```python
from build123d import *

# Parameters (mm, degrees)
SKETCH1_W                        = 82.55
SKETCH1_H                        = 127
EXTRUDE1_DEPTH                   = 12.7
SKETCH2_W                        = 57.15
SKETCH2_H                        = 127
CUT_EXTRUDE1_DEPTH               = 1.016
CUT_EXTRUDE2_REACH               = 14.7
SKETCH4_W                        = 12.7
SKETCH4_H                        = 127
EXTRUDE3_DEPTH                   = 107.95
EXTRUDE4_DEPTH                   = 12.7
CUT_EXTRUDE3_REACH               = 97.25
CUT_EXTRUDE4_DEPTH               = 96.25
F_1_2_13_TAPPED_HOLE1_AT_2_COUNT = 2
F_1_2_13_TAPPED_HOLE1_AT_2_PITCH = 34.925
F_1_2_13_TAPPED_HOLE2_AT_2_COUNT = 2
F_1_2_13_TAPPED_HOLE2_AT_2_PITCH = 44.45
FILLET1_R                        = 6.35
F_1_2_13_TAPPED_HOLE3_AT_2_COUNT = 2
F_1_2_13_TAPPED_HOLE3_AT_2_PITCH = 34.925
F_1_2_13_TAPPED_HOLE4_AT_2_COUNT = 2
F_1_2_13_TAPPED_HOLE4_AT_2_PITCH = 44.45


with BuildPart() as part:
    # Sketch1 → Extrude1 (new body)
    with BuildSketch(Plane.XY):
        with Locations((-41.275, 63.5)):
            Rectangle(SKETCH1_W, SKETCH1_H)
    extrude(amount=EXTRUDE1_DEPTH)

    # Sketch2 → Cut-Extrude1 (cut)
    with BuildSketch(Plane(origin=(0, 0, 0), x_dir=(-1, 0, 0), z_dir=(0, 0, -1))):
        with Locations((41.275, 63.5)):
            Rectangle(SKETCH2_W, SKETCH2_H)
    extrude(amount=-CUT_EXTRUDE1_DEPTH, mode=Mode.SUBTRACT)

    # Sketch3 → Cut-Extrude2 (cut, up to next)
    with BuildSketch(Plane.XY.offset(12.7), mode=Mode.PRIVATE) as cut_extrude2_sk1:
        with BuildLine():
            Line((-47.625, 114.935), (-34.925, 114.935))
            ThreePointArc((-34.925, 114.935), (-25.4, 105.41), (-34.925, 95.885))
            Line((-34.925, 95.885), (-47.625, 95.885))
            ThreePointArc((-47.625, 95.885), (-57.15, 105.41), (-47.625, 114.935))
        make_face()
    cut_extrude2_tool1 = extrude(cut_extrude2_sk1.sketch, amount=-CUT_EXTRUDE2_REACH, mode=Mode.PRIVATE) & part.part
    add(cut_extrude2_tool1.solids().sort_by_distance((-41.275, 105.41, 12.7))[0], mode=Mode.SUBTRACT)
    # Sketch3 → Cut-Extrude2 (cut, up to next)
    with BuildSketch(Plane.XY.offset(12.7), mode=Mode.PRIVATE) as cut_extrude2_sk2:
        with BuildLine():
            Line((-47.625, 31.115), (-34.925, 31.115))
            ThreePointArc((-34.925, 31.115), (-25.4, 21.59), (-34.925, 12.065))
            Line((-34.925, 12.065), (-47.625, 12.065))
            ThreePointArc((-47.625, 12.065), (-57.15, 21.59), (-47.625, 31.115))
        make_face()
    cut_extrude2_tool2 = extrude(cut_extrude2_sk2.sketch, amount=-CUT_EXTRUDE2_REACH, mode=Mode.PRIVATE) & part.part
    add(cut_extrude2_tool2.solids().sort_by_distance((-41.275, 21.59, 12.7))[0], mode=Mode.SUBTRACT)
    # Sketch3 → Cut-Extrude2 (cut, up to next)
    with BuildSketch(Plane.XY.offset(12.7), mode=Mode.PRIVATE) as cut_extrude2_sk3:
        with BuildLine():
            Line((-47.625, 76.835), (-34.925, 76.835))
            ThreePointArc((-34.925, 76.835), (-25.4, 67.31), (-34.925, 57.785))
            Line((-34.925, 57.785), (-47.625, 57.785))
            ThreePointArc((-47.625, 57.785), (-57.15, 67.31), (-47.625, 76.835))
        make_face()
    cut_extrude2_tool3 = extrude(cut_extrude2_sk3.sketch, amount=-CUT_EXTRUDE2_REACH, mode=Mode.PRIVATE) & part.part
    add(cut_extrude2_tool3.solids().sort_by_distance((-41.275, 67.31, 12.7))[0], mode=Mode.SUBTRACT)

    # Sketch4 → Extrude3 (add)
    with BuildSketch(Plane.XY.offset(12.7)):
        with Locations((-6.35, 63.5)):
            Rectangle(SKETCH4_W, SKETCH4_H)
    extrude(amount=EXTRUDE3_DEPTH)

    # Sketch5 → Extrude4 (add)
    with BuildSketch(Plane(origin=(0, 0, 0), x_dir=(0, 0, -1), z_dir=(1, 0, 0))):
        with BuildLine():
            Line((-120.65, 0), (-44.45, 0))
            Line((-44.45, 0), (-44.45, 299.085))
            Line((-44.45, 299.085), (-184.277, 299.085))
            Line((-184.277, 299.085), (-184.277, 149.86))
            Line((-184.277, 149.86), (-133.35, 149.86))
            ThreePointArc((-133.35, 149.86), (-124.369743879, 146.140256121), (-120.65, 137.16))
            Line((-120.65, 137.16), (-120.65, 0))
        make_face()
    extrude(amount=EXTRUDE4_DEPTH)

    # Sketch6 → Cut-Extrude3 (cut, up to next)
    with BuildSketch(Plane(origin=(12.7, 0, 0), x_dir=(0, 0, -1), z_dir=(1, 0, 0)), mode=Mode.PRIVATE) as cut_extrude3_sk1:
        Polygon((-127.127, 299.085), (-44.45, 127.635), (-44.45, 299.085), align=None)
    cut_extrude3_tool1 = extrude(cut_extrude3_sk1.sketch, amount=-CUT_EXTRUDE3_REACH, mode=Mode.PRIVATE) & part.part
    add(cut_extrude3_tool1.solids().sort_by_distance((12.7, 241.935, 72.009))[0], mode=Mode.SUBTRACT)

    # Sketch7 → Cut-Extrude4 (cut, through all)
    with BuildSketch(Plane(origin=(12.7, 0, 0), x_dir=(0, 0, -1), z_dir=(1, 0, 0))):
        Polygon((-184.277, 149.86), (-144.469555556, 149.86), (-184.277, 232.41), align=None)
    extrude(amount=-CUT_EXTRUDE4_DEPTH, mode=Mode.SUBTRACT)

    # Sketch8 → 1/2-13 Tapped Hole1 (revolve, cut)
    with BuildSketch(Plane(origin=(12.7, 248.285, 155.702), x_dir=(0, 0, -1), z_dir=(0, 1, 0))):
        Polygon((0, 0), (0, 12.7), (6.985, 12.7), (5.35813, 10.828500149), (5.35813, 1.871499851), (6.985, 0), align=None)
    f_1_2_13_tapped_hole1 = revolve(axis=Axis((19.05, 248.285, 155.702), (-1, 0, 0)), mode=Mode.SUBTRACT)

    # 1/2-13 Tapped Hole1 at 2: 1/2-13 Tapped Hole1 ×2
    with Locations(*[(0, i * F_1_2_13_TAPPED_HOLE1_AT_2_PITCH, 0) for i in range(1, F_1_2_13_TAPPED_HOLE1_AT_2_COUNT)]):
        add(f_1_2_13_tapped_hole1, mode=Mode.SUBTRACT)

    # Sketch10 → 1/2-13 Tapped Hole2 (revolve, cut)
    with BuildSketch(Plane(origin=(12.7, 210.185, 123.952), x_dir=(0, 0, -1), z_dir=(0, 1, 0))):
        Polygon((0, 0), (0, 12.7), (6.985, 12.7), (5.35813, 10.828500149), (5.35813, 1.871499851), (6.985, 0), align=None)
    f_1_2_13_tapped_hole2 = revolve(axis=Axis((19.05, 210.185, 123.952), (-1, 0, 0)), mode=Mode.SUBTRACT)

    # 1/2-13 Tapped Hole2 at 2: 1/2-13 Tapped Hole2 ×2
    with Locations(*[(0, -i * F_1_2_13_TAPPED_HOLE2_AT_2_PITCH, 0) for i in range(1, F_1_2_13_TAPPED_HOLE2_AT_2_COUNT)]):
        add(f_1_2_13_tapped_hole2, mode=Mode.SUBTRACT)

    # Fillet1
    fillet1_edges = [part.edges().sort_by_distance(p)[0] for p in [
        (-12.7, 63.5, 12.7),
    ]]
    fillet(fillet1_edges, radius=FILLET1_R)

    # Sketch16 → 1/2-13 Tapped Hole3 (revolve, cut)
    with BuildSketch(Plane(origin=(-95.25, 283.21, 155.702), x_dir=(0, 0, 1), z_dir=(0, 1, 0))):
        Polygon((0, 0), (0, 12.7), (6.985, 12.7), (5.35813, 10.828500149), (5.35813, 1.871499851), (6.985, 0), align=None)
    f_1_2_13_tapped_hole3 = revolve(axis=Axis((-101.6, 283.21, 155.702), (1, 0, 0)), mode=Mode.SUBTRACT)

    # 1/2-13 Tapped Hole3 at 2: 1/2-13 Tapped Hole3 ×2
    with Locations(*[(0, -i * F_1_2_13_TAPPED_HOLE3_AT_2_PITCH, 0) for i in range(1, F_1_2_13_TAPPED_HOLE3_AT_2_COUNT)]):
        add(f_1_2_13_tapped_hole3, mode=Mode.SUBTRACT)

    # Sketch18 → 1/2-13 Tapped Hole4 (revolve, cut)
    with BuildSketch(Plane(origin=(-95.25, 210.185, 123.952), x_dir=(0, 0, 1), z_dir=(0, 1, 0))):
        Polygon((0, 0), (0, 12.7), (6.985, 12.7), (5.35813, 10.828500149), (5.35813, 1.871499851), (6.985, 0), align=None)
    f_1_2_13_tapped_hole4 = revolve(axis=Axis((-101.6, 210.185, 123.952), (1, 0, 0)), mode=Mode.SUBTRACT)

    # 1/2-13 Tapped Hole4 at 2: 1/2-13 Tapped Hole4 ×2
    with Locations(*[(0, -i * F_1_2_13_TAPPED_HOLE4_AT_2_PITCH, 0) for i in range(1, F_1_2_13_TAPPED_HOLE4_AT_2_COUNT)]):
        add(f_1_2_13_tapped_hole4, mode=Mode.SUBTRACT)


solid = part.part
```
Could you check a few things on this model? Use its own coordinates, in mm. A direction names the side the tool comes from. Round coordinates to 2 decimals unless told otherwise and drop trailing zeros. Loops run counter-clockwise (first coordinate to the right, second up) from the corner with the lowest first, then second, coordinate; pieces in that order, holes last. Notation, with made-up numbers: M 38,-10.75 L 76,-10.75 A12 ccw 76,9.25 Z; hole C -15.5,68 d10. An arc over 180 degrees is marked long. Answer as CSV lines item,"result".
1) Imagine slicing it at D-D on y = 24. List the corners of the cut face in (x, z) for me, and give its area (3 significant figures).
From the geometry:
outline,"M -82.55,0 L -69.85,0 L -69.85,1.02 L -56.84,1.02 L -56.84,12.7 L -82.55,12.7 Z; M -25.71,1.02 L -12.7,1.02 L -12.7,0 L 0,0 L 0,44.45 L 12.7,44.45 L 12.7,120.65 L -12.7,120.65 L -12.7,19.05 A6.35 cw -19.05,12.7 L -25.71,12.7 Z"
area,"2,970 mm^2"
2) Imagine slicing it at A-A on y = 67.31. List the corners of the cut face in (x, z) for me, and give its area (3 significant figures).
From the geometry:
outline,"M -82.55,0 L -69.85,0 L -69.85,1.02 L -57.15,1.02 L -57.15,12.7 L -82.55,12.7 Z; M -25.4,1.02 L -12.7,1.02 L -12.7,0 L 0,0 L 0,44.45 L 12.7,44.45 L 12.7,120.65 L -12.7,120.65 L -12.7,19.05 A6.35 cw -19.05,12.7 L -25.4,12.7 Z"
area,"2,970 mm^2"
3) If I drill on probe 1 along X at (y, z) = (171.5, 74.5); probe 2 along X at (y, z) = (18.5, 80); probe 3 along Z at (x, y) = (-60, 78.5), over which ranges is the centre line in solid material (lowest first)?
From the geometry:
probe 1,"0 to 12.7"
probe 2,"-12.7 to 12.7"
probe 3,"1.02 to 12.7"
4) We'd pull the mould along Y, two halves only. Please class faces 4 (the flat face through (-3, 0, 52)), 5 (the cylindrical face through (6.41, 208.58, 118.84)), 6 (the cylindrical face through (-25.4, 105.6, 6.9)), 7 (the flat face through (0, 70, 120.65)): released by +Y, released by -Y, zero draft, split by the parting line, or undercut.
From the geometry:
face 4,"released by -Y"
face 5,"undercut"
face 6,"undercut"
face 7,"zero draft"
5) Imagine slicing it at B-B on x = -41. List the corners of the cut face in (y, z) for me (3 decimals).
From the geometry:
outline,"M 0,1.016 L 12.065,1.016 L 12.065,12.7 L 0,12.7 Z; M 31.115,1.016 L 57.785,1.016 L 57.785,12.7 L 31.115,12.7 Z; M 76.835,1.016 L 95.885,1.016 L 95.885,12.7 L 76.835,12.7 Z; M 114.935,1.016 L 127,1.016 L 127,12.7 L 114.935,12.7 Z"
6) Imagine slicing it at C-C on z = 138. List the corners of the cut face in (x, y) for me (3 decimals).
From the geometry:
outline,"M 0,149.86 L 12.7,149.86 L 12.7,299.085 L 0,299.085 Z"
7) For pin 1 Ø1 at (y, z) = (206, 112) entering from -X; pin 2 Ø6 at (x, y) = (-9, 78.5) entering from +Z; pin 3 Ø9.5 at (x, z) = (-39, 8.5) entering from +Y, each with a flat end and sliding along its axis, tell me the tip position at first contact or that it passes through.
From the geometry:
pin 1,"x = 0"
pin 2,"z = 120.65"
pin 3,"y = 127"
8) Which directions (+Z, -Z, +X, -X, +Y, -Y) give clear straight access to the entire face, cutting with the end or side of a thin tool? Please do faces 1 (the cylindrical face through (6.413, 167.787, 119.002)), 2 (the flat face through (-41, 76.835, 7)), 3 (the flat face through (6, 63, 44.45)).
From the geometry:
face 1,"+X, -X"
face 2,"+Z, -Z"
face 3,"-Z, +X, +Y, -Y"
